Geometry: final body of the model. Coordinates: model frame, mm. A direction names the side the tool comes from. Coordinates: 2 decimals unless noted, no trailing zeros. Loops run counter-clockwise (first coordinate to the right, second up) from the corner with the lowest first, then second, coordinate; pieces in that order, holes last. Notation, with made-up numbers: (-16, -14) -> (22, -14) arc R31 cw to (22, 21) -> close; hole circle Ø7 at (76.25, 71.25). An arc over 180 degrees is marked (long way). One line per item, written item: value. Start each with the question number.
Item 1: Section query A-A on y = 9.5. Return loops of the section in (x, z), then the cut area to 3 significant figures.
Item 2: Contact query for flat-ended pins moving along their axis: pin 1 Ø1.5 at (y, z) = (2.5, -2.5) entering from -X; pin 2 Ø3 at (y, z) = (10, -4) entering from -X; pin 3 Ø4 at (x, z) = (0, 0) entering from -Y; pin 4 Ø1.5 at (y, z) = (4.5, 7.5) entering from -X. Output: stop coordinate, or through.
Item 3: Ray query, probe 1 along Z at (x, y) = (0, -0.2); probe 2 along Y at (x, z) = (0.75, 8.5); probe 3 along Z at (x, y) = (0, 2.5). Return the intervals inside material, ascending. Write a range as from..to.
Item 4: Mould query, pull axis X, two halves, no side actions, for faces 1 (the cylindrical face through (-5.786, -0.246, 5.305)), 2 (the flat face through (-8, 0, 2)), 3 (the cylindrical face through (-4.864, 0.007, 4.461)). Classes: +X half, -X half, draft (parallel to the pull), parting line (faces both ways), or undercut.
Item 5: Set-up query: faces 4 (the flat face through (2, 0, 2)), 5 (the cylindrical face through (-0.54, 5.42, -2.44)), 6 (the flat face through (2, 11, 2)). Return all of +Z, -Z, +X, -X, +Y, -Y with unobstructed straight access to the full face (end or side cutting, diameter ignored); none if empty.
from build123d import *

# Parameters (mm, degrees)
SKETCH1_R                = 12
BOSS_EXTRUDE1_DEPTH      = 11
CHAMFER1_SIZE            = 2.7
SKETCH2_R                = 2.5
CUT_EXTRUDE1_DEPTH       = 12
SKETCH3_R                = 7.85
SKETCH3_R_2              = 6.6
BOSS_EXTRUDE4_DEPTH      = 0.5
BOSS_EXTRUDE4_DEPTH_BACK = 11.5
SKETCH3_4_R              = 6.6
SKETCH3_4_R_2            = 4.5
CUT_EXTRUDE2_DEPTH       = 0.5
CUT_EXTRUDE3_START       = -10.5
SKETCH3_5_R              = 6.6
SKETCH3_5_R_2            = 4.5
CUT_EXTRUDE3_DEPTH       = 0.5


with BuildPart() as part:
    # Sketch1 → Boss-Extrude1 (new body)
    with BuildSketch(Plane(origin=(0, 0, 0), x_dir=(1, 0, 0), z_dir=(0, 1, 0))):
        Circle(SKETCH1_R)
    extrude(amount=BOSS_EXTRUDE1_DEPTH)

    # Chamfer1
    chamfer1_edges = [part.edges().sort_by_distance(p)[0] for p in [
        (-12, 0, 0),
        (-12, 11, 0),
    ]]
    chamfer(chamfer1_edges, length=CHAMFER1_SIZE)

    # Sketch2 → Cut-Extrude1 (cut, through all)
    with BuildSketch(Plane.XZ):
        Circle(SKETCH2_R)
    extrude(amount=-CUT_EXTRUDE1_DEPTH, mode=Mode.SUBTRACT)

    # Sketch3 → Boss-Extrude4 (add, two sides)
    with BuildSketch(Plane.XZ) as boss_extrude4_sk:
        Circle(SKETCH3_R)
        Circle(SKETCH3_R_2, mode=Mode.SUBTRACT)
    extrude(amount=BOSS_EXTRUDE4_DEPTH)
    extrude(boss_extrude4_sk.sketch, amount=-BOSS_EXTRUDE4_DEPTH_BACK)

    # Sketch3_4 → Cut-Extrude2 (cut)
    with BuildSketch(Plane.XZ):
        Circle(SKETCH3_4_R)
        Circle(SKETCH3_4_R_2, mode=Mode.SUBTRACT)
    extrude(amount=-CUT_EXTRUDE2_DEPTH, mode=Mode.SUBTRACT)

    # Sketch3_5 → Cut-Extrude3 (cut)
    with BuildSketch(Plane.XZ.offset(CUT_EXTRUDE3_START)):
        Circle(SKETCH3_5_R)
        Circle(SKETCH3_5_R_2, mode=Mode.SUBTRACT)
    extrude(amount=-CUT_EXTRUDE3_DEPTH, mode=Mode.SUBTRACT)


solid = part.part
Reply:
1. outline: circle Ø21.6 at (0, 0); hole circle Ø5 at (0, 0)
1. area: 347 mm²
2. pin 1: stops at x = -11.87
2. pin 2: stops at x = -11.18
2. pin 3: passes through
2. pin 4: stops at x = -9.92
3. probe 1: z = -7.85..-6.6, 6.6..7.85
3. probe 2: y = 0..11
3. probe 3: z = -11.8..-2.5, 2.5..11.8
4. face 1: parting line
4. face 2: draft
4. face 3: undercut
5. face 4: -Y
5. face 5: +Y, -Y
5. face 6: +Y
